Autodesk Fusion 360 part; units mm, degrees
sketch "Sketch1" plane through (0, 0, 0) normal (0, 1, 0) x (1, 0, 0)
  line L0 (100, -50) -> (-100, -50)
  line L1 (-100, -50) -> (-100, 50)
  line L2 (-100, 50) -> (100, 50)
  line L3 (100, 50) -> (100, -50)
  line L4 (100, -50) -> (-100, 50) construction
  line L5 (-100, -50) -> (100, 50) construction
  line L6 (65, -25) -> (-65, -25)
  line L7 (-75, -15) -> (-75, 15)
  line L8 (-65, 25) -> (65, 25)
  line L9 (75, 15) -> (75, -15)
  line L10 (75, -25) -> (-75, 25) construction
  line L11 (-75, -25) -> (75, 25) construction
  circle A0 centre (0, 0) radius 12.5
  arc A1 (-65, 25) -> (-75, 15) centre (-65, 15) ccw
  arc A2 (-75, -15) -> (-65, -25) centre (-65, -15) ccw
  arc A3 (65, -25) -> (75, -15) centre (65, -15) ccw
  arc A4 (75, 15) -> (65, 25) centre (65, 15) ccw
  dimension "d1" = 200
  dimension "d2" = 100
  dimension "d3" = 150
  dimension "d4" = 50
  dimension "d5" = 25
  dimension "d6" = 10
extrude "Extrude1" add sketch "Sketch1" along normal blind 25 contours L0 L1 L2 L3
extrude "Extrude2" add sketch "Sketch1" along normal blind 10 contours L6 L7 L8 L9 A1 A2 A3 A4
extrude "Extrude3" add sketch "Sketch1" along normal blind 20 contours A0
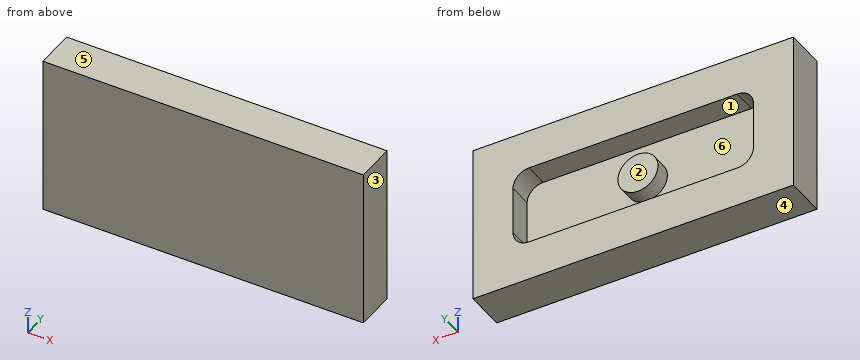
Read the model definition and answer for the solid it produces. Units are mm, in the model's axes. Face numbers are marked on the shaded views. A direction names the side the tool comes from. Round coordinates to 2 decimals unless told otherwise and drop trailing zeros. Write each loop counter-clockwise with the first axis right and the second up, starting at its lowest first coordinate (ties: lowest second). Pieces come first, ordered by that corner, then holes.
1. Given pin 1 Ø15 at (x, z) = (-21, -8.5) entering from +Y; pin 2 Ø1 at (x, z) = (-55.5, -30.5) entering from -Y, each flat-ended and moving along its own axis, determine where each tip first touches the part or whether it passes through.
2. Which of the six approach directions +Z, -Z, +X, -X, +Y, -Y give full straight-line access (tool end or side, diameter ignored) to the marked faces 5 and 6?
3. The part is cut by section D-D, the plane x = 0. Determine the outline of the cut face in (y, z), then the cut area to 3 significant figures.
4. The part is cut by section A-A, the plane y = 17.5. Determine the outline of the cut face in (x, z), then the cut area to 3 significant figures.
5. Determine the mould class of the marked faces 1, 2, 3 and 4 for opening direction X: pulls with the +X half, pulls with the -X half, needs draft (parallel to the pull), parting line crosses it, or undercut.
6. Straight lines are drawn through the part: L1, parallel to X at y = 11, z = -1; L2, parallel to X at y = 15.75, z = -13; L3, parallel to Z at x = 14, y = 20.5. For each, find the intervals that lie inside material, in ascending order.
7. The part is cut by section C-C, the plane x = 26.5. Determine the outline of the cut face in (y, z).
8. The part is cut by section B-B, the plane z = 10. Determine the outline of the cut face in (x, y), then the cut area to 3 significant figures.
Values:
1. pin 1: stops at y = 10
1. pin 2: stops at y = 0
2. face 5: +Z, +X, -X, +Y, -Y
2. face 6: +Y
3. outline: (0, -50) - (25, -50) - (25, -25) - (10, -25) - (10, -12.5) - (20, -12.5) - (20, 12.5) - (10, 12.5) - (10, 25) - (25, 25) - (25, 50) - (0, 50) - close
3. area: 2,000 mm2
4. outline: (-100, -50) - (100, -50) - (100, 50) - (-100, 50) - close; circle Ø25 at (0, 0); hole (-75, -15) arc R10 ccw to (-65, -25) - (65, -25) arc R10 ccw to (75, -15) - (75, 15) arc R10 ccw to (65, 25) - (-65, 25) arc R10 ccw to (-75, 15) - close
4. area: 13,100 mm2
5. face 1: undercut
5. face 2: undercut
5. face 3: pulls with the +X half
5. face 4: needs draft
6. L1: x = -100 to -75, -12.46 to 12.46, 75 to 100
6. L2: x = -100 to -75, 75 to 100
6. L3: z = -50 to -25, 25 to 50
7. outline: (0, -50) - (25, -50) - (25, -25) - (10, -25) - (10, 25) - (25, 25) - (25, 50) - (0, 50) - close
8. outline: (-100, 0) - (100, 0) - (100, 25) - (75, 25) - (75, 10) - (7.5, 10) - (7.5, 20) - (-7.5, 20) - (-7.5, 10) - (-75, 10) - (-75, 25) - (-100, 25) - close
8. area: 2,900 mm2
